from build123d import *

# Parameters (mm, degrees)
F0_W     = 76.2
F0_H     = 50.8
F1_DEPTH = 69.85
F2_W     = 63.605074
F2_H     = 13.815801
F2_W_2   = 63.892879
F2_H_2   = 12.952317
F2_W_3   = 62.741656
F2_H_3   = 8.922708
F3_DEPTH = 25.4


with BuildPart() as f1:
    # F0 (on Top) → F1 (new body)
    with BuildSketch(Plane.XY):
        with Locations((2.839793, 2.958526)):
            Rectangle(F0_W, F0_H)
    extrude(amount=F1_DEPTH)

    # F2 (on Front) → F3 (join)
    with BuildSketch(Plane.XZ):
        with Locations((3.456326, 54.260583)):
            Rectangle(F2_W, F2_H)
        with Locations((3.600228, 30.802497)):
            Rectangle(F2_W_2, F2_H_2)
        with Locations((3.024617, 10.078791)):
            Rectangle(F2_W_3, F2_H_3)
    extrude(amount=F3_DEPTH)


solid = f1.part
Here's how the part is built. I have some questions about the finished solid (model axes, mm). A direction names the side the tool comes from. Coordinates: 2 decimals unless noted, no trailing zeros. Order: outer loops, then holes, each group sorted by start corner. A loop starts at its lowest first (then second) coordinate and runs counter-clockwise, first axis right, second up. Notation, with made-up numbers: M 79,37.5 L 126,37.5 A14 cw 126,54.5 Z; hole C 74,87 d1. An arc over 180 degrees is marked long. Answer as CSV lines item,"result".
Item 1: If I drill on line 1 (Y direction, x = -11.5, z = 41), over which ranges is the centre line in solid material (lowest first)?
Results found:
line 1,"-22.44 to 28.36"
Item 2: Imagine slicing it at A-A on x = -26. Write out the boundary of the cut face in (y, z), plus the area to 3 significant figures.
Results found:
outline,"M -25.4,5.62 L -22.44,5.62 L -22.44,0 L 28.36,0 L 28.36,69.85 L -22.44,69.85 L -22.44,61.17 L -25.4,61.17 L -25.4,47.35 L -22.44,47.35 L -22.44,37.28 L -25.4,37.28 L -25.4,24.33 L -22.44,24.33 L -22.44,14.54 L -25.4,14.54 Z"
area,"3,650 mm2"
Item 3: For pin 1 (2.5 mm diameter, centred on y = -24.5, z = 10.5, fed in from +X); pin 2 (3.5 mm diameter, centred on x = 16, y = -24.5, fed in from +Z); pin 3 (0.9 mm diameter, centred on x = 18, y = -23.5, fed in from -Z), each with a flat end and sliding along its axis, tell me the tip position at first contact or that it passes through.
Results found:
pin 1,"x = 34.4"
pin 2,"z = 61.17"
pin 3,"z = 5.62"
Item 4: We'd pull the mould along Z, two halves only. Please class faces 4 (the face through (2, 3, 0)), 5 (the face through (35.259, -24, 54)), 6 (the face through (3, -24, 14.54)), 7 (the face through (3, -24, 24.326)): +Z half, -Z half, draft (parallel to the pull), parting line (faces both ways), or undercut.
Results found:
face 4,"-Z half"
face 5,"draft"
face 6,"undercut"
face 7,"undercut"
Item 5: On a 3-axis mill with a long thin cutter (end or side, diameter ignored), from which of +Z, -Z, +X, -X, +Y, -Y can I reach the whole of each face in a straight line? I mean faces 1 (the face through (3, -24, 5.617)), 2 (the face through (3, -24, 47.353)), 3 (the face through (-28.346, -24, 10)). Say none if no direction works.
Results found:
face 1,"-Z, +X, -X, -Y"
face 2,"+X, -X, -Y"
face 3,"+Z, -Z, -X, -Y"
Item 6: Imagine slicing it at B-B on z = 62.5. Write out the boundary of the cut face in (x, y).
Results found:
outline,"M -35.26,-22.44 L 40.94,-22.44 L 40.94,28.36 L -35.26,28.36 Z"
